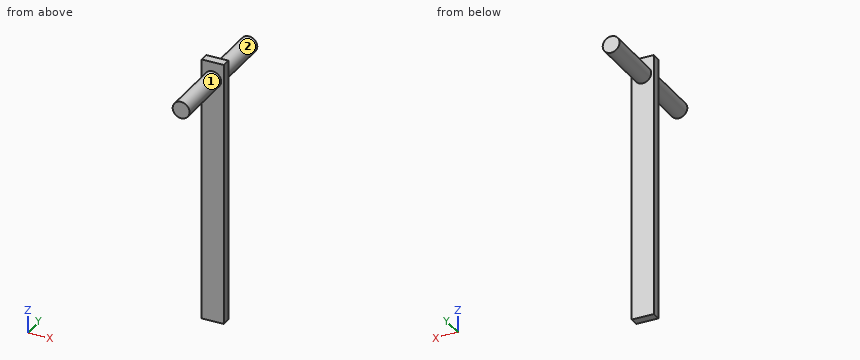
```python
from build123d import *

# Parameters (mm, degrees)
F0_W     = 12.7
F0_H     = 5.08
F1_DEPTH = 76.2
F2_R     = 4.826
F3_DEPTH = 38.1


with BuildPart() as f1:
    # F0 (on Top) → F1 (new body, symmetric)
    with BuildSketch(Plane.XY):
        Rectangle(F0_W, F0_H)
    extrude(amount=F1_DEPTH, both=True)

    # F2 (on Front) → F3 (join, symmetric)
    with BuildSketch(Plane.XZ):
        with Locations((0, 66.04)):
            Circle(F2_R)
    extrude(amount=F3_DEPTH, both=True)


solid = f1.part
```
Geometry check sheet. Reference: the model listing, model coordinates, mm. Face numbers are marked on the shaded views. A direction names the side the tool comes from. Coordinates: 2 decimals unless noted, no trailing zeros. Order: outer loops, then holes, each group sorted by start corner. A loop starts at its lowest first (then second) coordinate and runs counter-clockwise, first axis right, second up. Notation, with made-up numbers: (36, -39) - (71, -39) arc R4 ccw to (71, -33) - close; hole circle Ø8 at (-39, 54.5). An arc over 180 degrees is marked (long way). Use one line per item in the form item = value.
1. Section check C-C (y = -29). Record the boundary of the cut face in (x, z), then the cut area to 3 significant figures.
Here are the results:
outline = circle Ø9.65 at (0, 66.04)
area = 73.2 mm²
2. Section check A-A (x = 0). Record the boundary of the cut face in (y, z).
Here are the results:
outline = (-38.1, 61.21) - (-2.54, 61.21) - (-2.54, -76.2) - (2.54, -76.2) - (2.54, 61.21) - (38.1, 61.21) - (38.1, 70.87) - (2.54, 70.87) - (2.54, 76.2) - (-2.54, 76.2) - (-2.54, 70.87) - (-38.1, 70.87) - close
3. Scan lines: line 1 (X direction, y = 24, z = 66); line 2 (Z direction, x = 0, y = 30.5); line 3 (Y direction, x = -0.25, z = 45). Record each from-to range of solid material in increasing order.
Here are the results:
line_1 = -4.83 to 4.83
line_2 = 61.21 to 70.87
line_3 = -2.54 to 2.54
4. Access from +Z, -Z, +X, -X, +Y, -Y to the whole of each face (thin tool, end or side, straight path). Record for the marked faces 1 and 2.
Here are the results:
face_1 = -Y
face_2 = +Y
5. Section check D-D (z = -24). Record the boundary of the cut face in (x, y), then the cut area to 3 significant figures.
Here are the results:
outline = (-6.35, -2.54) - (6.35, -2.54) - (6.35, 2.54) - (-6.35, 2.54) - close
area = 64.5 mm²
6. Section check B-B (z = 66.04). Record the boundary of the cut face in (x, y).
Here are the results:
outline = (-6.35, -2.54) - (-4.83, -2.54) - (-4.83, -38.1) - (4.83, -38.1) - (4.83, -2.54) - (6.35, -2.54) - (6.35, 2.54) - (4.83, 2.54) - (4.83, 38.1) - (-4.83, 38.1) - (-4.83, 2.54) - (-6.35, 2.54) - close
7. Gauge pin test, flat ends, axial feed: pin 1 (4 mm diameter, centred on x = 1.5, z = -35.5, fed in from +Y); pin 2 (2 mm diameter, centred on x = -2, z = 18, fed in from -Y); pin 3 (3 mm diameter, centred on x = 0.5, y = 9.5, fed in from +Z). Record the tip position at first contact, or that the pin passes through.
Here are the results:
pin_1 = 2.54
pin_2 = -2.54
pin_3 = 70.87
